from build123d import *

# Parameters (mm, degrees)
SKETCH1_W           = 40
SKETCH1_H           = 20
SKETCH1_R           = 2
BOSS_EXTRUDE1_DEPTH = 5
SKETCH2_W           = 19.5
SKETCH2_H           = 6.5
CUT_EXTRUDE1_DEPTH  = 3.25


with BuildPart() as part:
    # Sketch1 → Boss-Extrude1 (new, symmetric)
    with BuildSketch(Plane(origin=(0, 0, 0), x_dir=(1, 0, 0), z_dir=(0, 1, 0))):
        Rectangle(SKETCH1_W, SKETCH1_H)
        with Locations(Location((-16, 6, 0), (0, 0, 270))):
            Circle(SKETCH1_R, mode=Mode.SUBTRACT)
        with Locations(Location((16, 6, 0), (0, 0, 270))):
            Circle(SKETCH1_R, mode=Mode.SUBTRACT)
        with Locations(Location((16, -6, 0), (0, 0, 270))):
            Circle(SKETCH1_R, mode=Mode.SUBTRACT)
        with Locations(Location((-16, -6, 0), (0, 0, 270))):
            Circle(SKETCH1_R, mode=Mode.SUBTRACT)
    extrude(amount=BOSS_EXTRUDE1_DEPTH, both=True)

    # Sketch2 → Cut-Extrude1 (cut, symmetric)
    with BuildSketch(Plane(origin=(0, 5, 0), x_dir=(1, 0, 0), z_dir=(0, 1, 0))):
        Rectangle(SKETCH2_W, SKETCH2_H)
    cut_extrude1 = extrude(amount=CUT_EXTRUDE1_DEPTH, both=True, mode=Mode.SUBTRACT)

    # Mirror1: Cut-Extrude1 across plane
    add(cut_extrude1.mirror(Plane.ZX), mode=Mode.SUBTRACT)


solid = part.part
The listing builds one solid part. Answer for the finished solid, in the listing's coordinates (mm). A direction names the side the tool comes from. Coordinates: 2 decimals unless noted, no trailing zeros. Loops run counter-clockwise (first coordinate to the right, second up) from the corner with the lowest first, then second, coordinate; pieces in that order, holes last. Notation, with made-up numbers: M 34,-20 L 78,-20 A21 ccw 78,-1 Z; hole C -35,72.25 d9. An arc over 180 degrees is marked long. Answer in a Markdown table with one row per item.
1) Given pin 1 (2 mm diameter, centred on x = -6, z = 1.5, fed in from +Y); pin 2 (4.5 mm diameter, centred on x = 16, z = -6, fed in from -Y); pin 3 (3 mm diameter, centred on x = -5, z = 1.5, fed in from -Y), each flat-ended and moving along its own axis, determine where each tip first touches the part or whether it passes through.
Answers below:
| item | result |
|---|---|
| pin 1 | y = 1.75 |
| pin 2 | y = -5 |
| pin 3 | y = -1.75 |
2) Which of the six approach directions +Z, -Z, +X, -X, +Y, -Y give full straight-line access (tool end or side, diameter ignored) to faces 4 (the flat face through (0, 1.75, 0)), 5 (the flat face through (0, -1.75, 0)), 6 (the flat face through (0, -5, -5))?
Answers below:
| item | result |
|---|---|
| face 4 | +Y |
| face 5 | -Y |
| face 6 | +Z, -Z, +X, -X, -Y |
3) Find section A-A (y = 3.25). Determine the outline of the cut face in (x, z), then the cut area to 3 significant figures.
Answers below:
| item | result |
|---|---|
| outline | M -20,-10 L 20,-10 L 20,10 L -20,10 Z; hole C -16,-6 d4; hole C -16,6 d4; hole M -9.75,-3.25 L 9.75,-3.25 L 9.75,3.25 L -9.75,3.25 Z; hole C 16,-6 d4; hole C 16,6 d4 |
| area | 623 mm^2 |
4) Find section C-C (z = -6). Determine the outline of the cut face in (x, y).
Answers below:
| item | result |
|---|---|
| outline | M -20,-5 L -18,-5 L -18,5 L -20,5 Z; M -14,-5 L 14,-5 L 14,5 L -14,5 Z; M 18,-5 L 20,-5 L 20,5 L 18,5 Z |
5) Find the intervals of material crossed by probe 1 along X at (y, z) = (4, -6); probe 2 along X at (y, z) = (-2, -3); probe 3 along Z at (x, y) = (-17.5, 4.5), in increasing order.
Answers below:
| item | result |
|---|---|
| probe 1 | -20 to -18, -14 to 14, 18 to 20 |
| probe 2 | -20 to -9.75, 9.75 to 20 |
| probe 3 | -10 to -7.32, -4.68 to 4.68, 7.32 to 10 |
6) Find section D-D (x = -7). Determine the outline of the cut face in (y, z), then the cut area to 3 significant figures.
Answers below:
| item | result |
|---|---|
| outline | M -5,-10 L 5,-10 L 5,-3.25 L 1.75,-3.25 L 1.75,3.25 L 5,3.25 L 5,10 L -5,10 L -5,3.25 L -1.75,3.25 L -1.75,-3.25 L -5,-3.25 Z |
| area | 158 mm^2 |
7) Determine the mould class of faces 1 (the flat face through (0, 0, 10)), 2 (the flat face through (-20, 0, 0)), 3 (the cylindrical face through (-14, 0, -6)) for opening direction X: released by +X, released by -X, zero draft, split by the parting line, or undercut.
Answers below:
| item | result |
|---|---|
| face 1 | zero draft |
| face 2 | released by -X |
| face 3 | undercut |
8) Find section B-B (x = 16). Determine the outline of the cut face in (y, z).
Answers below:
| item | result |
|---|---|
| outline | M -5,-10 L 5,-10 L 5,-8 L -5,-8 Z; M -5,-4 L 5,-4 L 5,4 L -5,4 Z; M -5,8 L 5,8 L 5,10 L -5,10 Z |
